Geometry check sheet. Reference: the model listing, model coordinates, mm. A direction names the side the tool comes from. Coordinates: 2 decimals unless noted, no trailing zeros. Order: outer loops, then holes, each group sorted by start corner. A loop starts at its lowest first (then second) coordinate and runs counter-clockwise, first axis right, second up. Notation, with made-up numbers: (64.25, 0) - (79.25, 0) arc R5 ccw to (79.25, 9) - close; hole circle Ø1 at (78.25, -4). An arc over 180 degrees is marked (long way). Put each result on its own line as item: value.
Autodesk Inventor part; units mm, degrees
ref_plane "m1_XY" through (0, 5.5563, 0) normal (0, 0, 1) x (1, 0, 0)
ref_plane "m1_YZ" through (0, 5.5563, 0) normal (1, 0, 0) x (0, 1, 0)
ref_plane "m1_ZX" through (0, 5.5563, 0) normal (0, 1, 0) x (0, 0, 1)
sketch "Sketch_2" plane through (0, 0, 0) normal (0, 0, 1) x (1, 0, 0)
  line L0 (9.525, 0) -> (0, 0)
  line L1 (0, 0) -> (0, 4.8006)
  line L2 (0, 4.8006) -> (0.7557, 5.5563)
  line L3 (0.7557, 5.5563) -> (4.6603, 5.5563)
  line L4 (4.6603, 5.5563) -> (5.4159, 4.8006)
  line L5 (5.4159, 4.8006) -> (5.4788, 4.7498)
  arc A0 (5.4788, 4.7498) -> (5.9817, 4.572) centre (5.9817, 5.3721) ccw
  line L6 (5.9817, 4.572) -> (7.1501, 4.572)
  arc A1 (7.1501, 4.572) -> (7.9502, 5.3721) centre (7.1501, 5.3721) ccw
  line L7 (7.9502, 5.3721) -> (7.9502, 5.5309)
  line L8 (7.9502, 5.5309) -> (9.525, 5.5309)
  line L9 (9.525, 5.5309) -> (9.525, 0)
  line L10 (9.525, 0) -> (0, 0)
revolve "Revolution1" add sketch "Sketch_2" angle 360 about axis through (9.525, 0, 0) along (1, 0, 0)
thread "Thread1"
sketch "Sketch_3" plane through (0, 0, 0) normal (0, 0, 1) x (1, 0, 0)
  line L0 (29.3624, 0) -> (9.525, 0)
  line L1 (9.525, 0) -> (9.525, 7.0485)
  line L2 (9.525, 7.0485) -> (10.287, 7.8105)
  line L3 (10.287, 7.8105) -> (25.1206, 7.8105)
  line L4 (25.1206, 7.8105) -> (25.3746, 7.5565)
  line L5 (25.3746, 7.5565) -> (25.3746, 6.6357)
  line L6 (25.3746, 6.6357) -> (26.0096, 6.6357)
  line L7 (26.0096, 6.6357) -> (26.6446, 7.2708)
  line L8 (26.6446, 7.2708) -> (28.8544, 7.2708)
  line L9 (28.8544, 7.2708) -> (29.3624, 6.7627)
  line L10 (29.3624, 6.7627) -> (29.3624, 0)
  line L11 (29.3624, 0) -> (9.525, 0)
revolve "Revolution2" add sketch "Sketch_3" angle 360 about axis through (29.3624, 0, 0) along (1, 0, 0)
sketch "Sketch_12" plane through (0, 0, 0) normal (0, 1, 0) x (-1, 0, 0)
  line L0 (-19.05, 7.8105) -> (-19.05, -1.016)
  line L1 (-19.05, -1.016) -> (-21.0337, -1.016)
  line L2 (-21.0337, -1.016) -> (-21.0337, 6.3652)
  line L3 (-21.0337, 6.3652) -> (-21.463, 6.7945)
  line L4 (-21.463, 6.7945) -> (-23.0124, 6.7945)
  line L5 (-23.0124, 6.7945) -> (-23.0124, 7.8105)
  line L6 (-23.0124, 7.8105) -> (-19.05, 7.8105)
  line L7 (-19.05, 7.8105) -> (-19.05, -1.016)
revolve "Revolution3" cut sketch "Sketch_12" angle 360 about axis through (19.05, 0, 7.8105) along (0, 0, 1)
thread "Thread2"
sketch "Sketch_47" plane through (0, 0, 0) normal (0, 0, 1) x (1, 0, 0)
  line L0 (26.0096, 0) -> (25.3746, 0)
  line L1 (25.3746, 6.3818) -> (26.0096, 6.3818)
  line L2 (26.0096, 6.3818) -> (26.0096, 6.6357)
  line L3 (26.0096, 6.6357) -> (25.6921, 6.6357)
  line L4 (25.6921, 6.6357) -> (25.4916, 6.8362)
  arc A0 (25.4916, 7.0158) -> (25.4916, 6.8362) centre (25.5814, 6.926) ccw
  line L5 (25.4916, 7.0158) -> (26.2022, 7.7263)
  line L6 (26.2022, 7.7263) -> (26.2022, 7.8105)
  line L7 (26.2022, 7.8105) -> (25.999, 7.8105)
  line L8 (25.999, 7.8105) -> (25.3746, 7.1861)
  line L9 (25.3746, 7.1861) -> (25.3746, 6.3818)
revolve "Revolution4" add sketch "Sketch_47" angle 360 about axis through (26.0096, 0, 0) along (1, 0, 0)
sketch "Sketch_33" plane through (0, 0, 0) normal (1, 0, 0) x (0, 1, 0)
  line L0 (1.778, 2.794) -> (-1.778, 2.794)
  arc A0 (-1.778, 2.794) -> (-2.794, 1.778) centre (-1.778, 1.778) ccw
  line L1 (-2.794, 1.778) -> (-2.794, -1.778)
  arc A1 (-2.794, -1.778) -> (-1.778, -2.794) centre (-1.778, -1.778) ccw
  line L2 (-1.778, -2.794) -> (1.778, -2.794)
  arc A2 (1.778, -2.794) -> (2.794, -1.778) centre (1.778, -1.778) ccw
  line L3 (2.794, -1.778) -> (2.794, 1.778)
  arc A3 (2.794, 1.778) -> (1.778, 2.794) centre (1.778, 1.778) ccw
extrude "Extrusion1" cut sketch "Sketch_33" along normal blind 58.7248
ref_plane "m1_XY" through (0, 5.5563, 0) normal (0, 0, 1) x (1, 0, 0)
ref_plane "m1_YZ" through (0, 5.5563, 0) normal (1, 0, 0) x (0, 1, 0)
ref_plane "m1_ZX" through (0, 5.5563, 0) normal (0, 1, 0) x (0, 0, 1)
ref_plane "m2_XY" through (0, -5.5563, 0) normal (0, 0, 1) x (1, 0, 0)
ref_plane "m2_YZ" through (0, -5.5563, 0) normal (1, 0, 0) x (0, 1, 0)
ref_plane "m2_ZX" through (0, -5.5563, 0) normal (0, 1, 0) x (0, 0, 1)
ref_plane "s1_XY" through (7.9502, 0, 0) normal (0, 0, 1) x (1, 0, 0)
ref_plane "s1_YZ" through (7.9502, 0, 0) normal (1, 0, 0) x (0, 1, 0)
ref_plane "s1_ZX" through (7.9502, 0, 0) normal (0, 1, 0) x (0, 0, 1)
ref_plane "s2_XY" through (9.525, 0, 0) normal (0, 0, 1) x (1, 0, 0)
ref_plane "s2_YZ" through (9.525, 0, 0) normal (1, 0, 0) x (0, 1, 0)
ref_plane "s2_ZX" through (9.525, 0, 0) normal (0, 1, 0) x (0, 0, 1)
ref_plane "dp1_XY" through (9.525, 5.5309, 0) normal (0, 0, 1) x (1, 0, 0)
ref_plane "dp1_YZ" through (9.525, 5.5309, 0) normal (1, 0, 0) x (0, 1, 0)
ref_plane "dp1_ZX" through (9.525, 5.5309, 0) normal (0, 1, 0) x (0, 0, 1)
ref_plane "dp2_XY" through (9.525, -5.5309, 0) normal (0, 0, 1) x (1, 0, 0)
ref_plane "dp2_YZ" through (9.525, -5.5309, 0) normal (1, 0, 0) x (0, 1, 0)
ref_plane "dp2_ZX" through (9.525, -5.5309, 0) normal (0, 1, 0) x (0, 0, 1)
ref_plane "rod_guide_XY" through (0, 0, 0) normal (1, 0, 0) x (0, 0, -1)
ref_plane "rod_guide_YZ" through (0, 0, 0) normal (0, 0, -1) x (0, 1, 0)
ref_plane "rod_guide_ZX" through (0, 0, 0) normal (0, 1, 0) x (1, 0, 0)
ref_plane "to_tube_XY" through (26.0096, 0, 0) normal (1, 0, 0) x (0, 0, -1)
ref_plane "to_tube_YZ" through (26.0096, 0, 0) normal (0, 0, -1) x (0, 1, 0)
ref_plane "to_tube_ZX" through (26.0096, 0, 0) normal (0, 1, 0) x (1, 0, 0)
ref_plane "to_foot_bracket_XY" through (9.525, 0, 0) normal (1, 0, 0) x (0, 0, -1)
ref_plane "to_foot_bracket_YZ" through (9.525, 0, 0) normal (0, 0, -1) x (0, 1, 0)
ref_plane "to_foot_bracket_ZX" through (9.525, 0, 0) normal (0, 1, 0) x (1, 0, 0)
ref_plane "to_nut_XY" through (9.525, 0, 0) normal (1, 0, 0) x (0, 0, -1)
ref_plane "to_nut_YZ" through (9.525, 0, 0) normal (0, 0, -1) x (0, 1, 0)
ref_plane "to_nut_ZX" through (9.525, 0, 0) normal (0, 1, 0) x (1, 0, 0)
ref_plane "to_trunnion_brackets_XY" through (0, 0, 0) normal (0, 1, 0) x (1, 0, 0)
ref_plane "to_trunnion_brackets_YZ" through (0, 0, 0) normal (1, 0, 0) x (0, 0, -1)
ref_plane "to_trunnion_brackets_ZX" through (0, 0, 0) normal (0, 0, -1) x (0, 1, 0)
ref_plane "to_trunnion_brackets1_XY" through (0, 0, 0) normal (0, 1, 0) x (1, 0, 0)
ref_plane "to_trunnion_brackets1_YZ" through (0, 0, 0) normal (1, 0, 0) x (0, 0, -1)
ref_plane "to_trunnion_brackets1_ZX" through (0, 0, 0) normal (0, 0, -1) x (0, 1, 0)
ref_plane "to_trunnion_brackets2_XY" through (0, 0, 0) normal (0, 1, 0) x (1, 0, 0)
ref_plane "to_trunnion_brackets2_YZ" through (0, 0, 0) normal (1, 0, 0) x (0, 0, -1)
ref_plane "to_trunnion_brackets2_ZX" through (0, 0, 0) normal (0, 0, -1) x (0, 1, 0)
ref_plane "t1_XY" through (9.525, 0, 0) normal (1, 0, 0) x (0, 0, -1)
ref_plane "t1_YZ" through (9.525, 0, 0) normal (0, 0, -1) x (0, 1, 0)
ref_plane "t1_ZX" through (9.525, 0, 0) normal (0, 1, 0) x (1, 0, 0)
ref_plane "port_XY" through (19.05, 0, 0) normal (0, 0, 1) x (1, 0, 0)
ref_plane "port_YZ" through (19.05, 0, 0) normal (1, 0, 0) x (0, 1, 0)
ref_plane "port_ZX" through (19.05, 0, 0) normal (0, 1, 0) x (0, 0, 1)
ref_plane "rod_guide_1_XY" through (0, 0, 0) normal (1, 0, 0) x (0, 0, -1)
ref_plane "rod_guide_1_YZ" through (0, 0, 0) normal (0, 0, -1) x (0, 1, 0)
ref_plane "rod_guide_1_ZX" through (0, 0, 0) normal (0, 1, 0) x (1, 0, 0)
ref_plane "rod_guide_11_XY" through (0, 0, 0) normal (1, 0, 0) x (0, 0, -1)
ref_plane "rod_guide_11_YZ" through (0, 0, 0) normal (0, 0, -1) x (0, 1, 0)
ref_plane "rod_guide_11_ZX" through (0, 0, 0) normal (0, 1, 0) x (1, 0, 0)
properties part number "02R0101_NR_rod_guide"
Q1. Access from +Z, -Z, +X, -X, +Y, -Y to the whole of each face (thin tool, end or side, straight path). Record for faces 4 (the cylindrical face through (14.48, -2.5, 2.49)), 5 (the cylindrical face through (27.765, -5.77, -4.424)), 6 (the flat face through (21, 2, 6.794)), 7 (the cylindrical face through (8.7, -1.2, -5.4)).
Answer block:
face 4: +X, -X
face 5: +X
face 6: +Z
face 7: none
Q2. Thickness scan on L1, parallel to Z at x = 4.25, y = -0.5; L2, parallel to X at y = 0, z = 3.7; L3, parallel to X at y = 0, z = 5.05. Record the ranges inside material, lowest first. Write a range as [from, to].
Answer block:
L1: z = [-5.53, -2.79], [2.79, 5.53]
L2: x = [0, 17.07], [21.03, 29.36]
L3: x = [0.25, 5.17], [7.88, 17.07], [21.03, 29.36]
Q3. Section check A-A on x = 14.5. Record the boundary of the cut face in (y, z), then the cut area to 3 significant figures.
Answer block:
outline: circle Ø15.62 at (0, 0); hole (-2.79, -1.78) arc R1.02 ccw to (-1.78, -2.79) - (1.78, -2.79) arc R1.02 ccw to (2.79, -1.78) - (2.79, 1.78) arc R1.02 ccw to (1.78, 2.79) - (-1.78, 2.79) arc R1.02 ccw to (-2.79, 1.78) - close
area: 161 mm^2
Q4. Section check D-D on x = 27.75. Record the boundary of the cut face in (y, z).
Answer block:
outline: circle Ø14.54 at (0, 0); hole (-2.79, -1.78) arc R1.02 ccw to (-1.78, -2.79) - (1.78, -2.79) arc R1.02 ccw to (2.79, -1.78) - (2.79, 1.78) arc R1.02 ccw to (1.78, 2.79) - (-1.78, 2.79) arc R1.02 ccw to (-2.79, 1.78) - close
Q5. Depth check by flat-ended pin: pin 1 Ø4 at (x, y) = (18.5, 0) entering from +Z; pin 2 Ø3 at (x, y) = (19.05, 0) entering from +Z; pin 3 Ø4 at (x, y) = (19, -2.5) entering from +Z. Enter the tip coordinate at first touch or a pass-through.
Answer block:
pin 1: stops at z = 6.79
pin 2: stops at z = -2.79
pin 3: stops at z = 6.95
Q6. Draft check along X on faces 1 (the flat face through (29.362, 3, 0)), 2 (the cylindrical face through (20.94, 0.6, 4.59)), 3 (the flat face through (14, 2.794, 0)). Enter one of: pulls with the +X half, pulls with the -X half, needs draft (parallel to the pull), parting line crosses it, or undercut.
Answer block:
face 1: pulls with the +X half
face 2: undercut
face 3: needs draft
Q7. Section check C-C on y = 0. State how many separate pieces and enclosed holes the cut face has, then the cut area to 3 significant figures.
Answer block:
separate pieces: 3
enclosed holes: 0
area: 216 mm^2
Q8. Section check B-B on x = 19.05. Record the boundary of the cut face in (y, z).
Answer block:
outline: (-3.85, 6.79) arc R7.81 ccw (long way) to (3.85, 6.79) - (2.41, 6.79) - (1.98, 6.37) - (1.98, 2.77) arc R1.02 cw to (2.79, 1.78) - (2.79, -1.78) arc R1.02 cw to (1.78, -2.79) - (-1.78, -2.79) arc R1.02 cw to (-2.79, -1.78) - (-2.79, 1.78) arc R1.02 cw to (-1.98, 2.77) - (-1.98, 6.37) - (-2.41, 6.79) - close
